Geometry check sheet. Reference: the model listing, model coordinates, mm. Coordinates: 2 decimals unless noted, no trailing zeros. Order: outer loops, then holes, each group sorted by start corner. A loop starts at its lowest first (then second) coordinate and runs counter-clockwise, first axis right, second up. Notation, with made-up numbers: M -15.75,53.5 L -1.75,53.5 A12 ccw -1.75,65.5 Z; hole C -3.75,36.25 d5. An arc over 180 degrees is marked long. One line per item, written item: value. Start each with the question number.
1) Go/stop test with flat-tipped pins: P1, Ø1.5, axis at y = 20, z = 3, coming from the +X side; P2, Ø1.5, axis at y = 99, z = 2, coming from the +X side (3 decimals); P3, Ø4.5, axis at x = -106, y = -70.5, coming from the +Z side. Record where each tip stops, or that it passes through.
2) Sectioned sample at D-D, the plane y = -207. Enter the section's corners in (x, z), then the cut area to 3 significant figures.
3) Thickness scan on L1, parallel to X at y = 81.5, z = 0.5; L2, parallel to Y at x = -1, z = 3.15; L3, parallel to X at y = -286.75, z = 1.15. Record the ranges inside material, lowest first. Write a range as from..to.
4) Sectioned sample at A-A, the plane y = -123. Enter the section's corners in (x, z).
5) Sectioned sample at C-C, the plane x = -61.5. Enter the section's corners in (y, z).
6) Sectioned sample at B-B, the plane z = 1.75. State how many separate pieces and enclosed holes the cut face has, then the cut area to 3 significant figures.
```python
from build123d import *

# Parameters (mm, degrees)
SKETCH1_R           = 2.75
BOSS_EXTRUDE1_DEPTH = 5
SKETCH2_R           = 3.25
BOSS_EXTRUDE2_DEPTH = 5
SKETCH3_R           = 2.75
BOSS_EXTRUDE3_DEPTH = 5
SKETCH4_R           = 3.25
BOSS_EXTRUDE4_DEPTH = 5
SKETCH5_R           = 2.75
BOSS_EXTRUDE5_DEPTH = 5
SKETCH6_R           = 3.25
BOSS_EXTRUDE6_DEPTH = 5


with BuildPart() as part:
    # Sketch1 → Boss-Extrude1 (new body)
    with BuildSketch(Plane.XY):
        Polygon((0, 210), (0, 0), (230, 0), (285, 210), align=None)
        with Locations((104, 185.5)):
            Circle(SKETCH1_R, mode=Mode.SUBTRACT)
        with Locations((194, 176)):
            Circle(SKETCH1_R, mode=Mode.SUBTRACT)
        with Locations((108.5, 130)):
            Circle(SKETCH1_R, mode=Mode.SUBTRACT)
        with Locations((193.5, 112)):
            Circle(SKETCH1_R, mode=Mode.SUBTRACT)
        with Locations((138.5, 82.5)):
            Circle(SKETCH1_R, mode=Mode.SUBTRACT)
        with Locations((167.5, 79.5)):
            Circle(SKETCH1_R, mode=Mode.SUBTRACT)
        with Locations((40, 83)):
            Circle(SKETCH1_R, mode=Mode.SUBTRACT)
        with Locations((66, 79)):
            Circle(SKETCH1_R, mode=Mode.SUBTRACT)
    extrude(amount=BOSS_EXTRUDE1_DEPTH)

    # Sketch2 → Boss-Extrude2 (add)
    with BuildSketch(Plane.XY):
        with BuildLine():
            Line((-202.121956495, 0), (0, 0))
            Line((0, 0), (0, 210))
            Line((0, 210), (-290, 210))
            Line((-290, 210), (-230, 0))
            Line((-230, 0), (-208.306614933, 0))
            ThreePointArc((-208.306614933, 0), (-205.214285714, 2.25), (-202.121956495, 0))
        make_face()
        with Locations((-237, 115.5)):
            Circle(SKETCH2_R, mode=Mode.SUBTRACT)
    extrude(amount=BOSS_EXTRUDE2_DEPTH)

    # Sketch3 → Boss-Extrude3 (add)
    with BuildSketch(Plane.XY):
        with BuildLine():
            Line((-208.306614933, 0), (-230, 0))
            Line((-230, 0), (-170, -210))
            Line((-170, -210), (-68.5, -210))
            Line((-68.5, -210), (-68.5, -81.5))
            Line((-68.5, -81.5), (0, -81.5))
            Line((0, -81.5), (0, -25.304886114))
            ThreePointArc((0, -25.304886114), (-4.25, -23), (0, -20.695113886))
            Line((0, -20.695113886), (0, 0))
            Line((0, 0), (-202.121956495, 0))
            ThreePointArc((-202.121956495, 0), (-202.003945393, -0.493823135), (-201.964285714, -1))
            ThreePointArc((-201.964285714, -1), (-205.720462579, -4.210340322), (-208.306614933, 0))
        make_face()
        with Locations((-106, -70.5)):
            Circle(SKETCH3_R, mode=Mode.SUBTRACT)
        with Locations((-93.5, -65.5)):
            Circle(SKETCH3_R, mode=Mode.SUBTRACT)
        with Locations((-4, -68.75)):
            Circle(SKETCH3_R, mode=Mode.SUBTRACT)
        with Locations((-105.75, -23.5)):
            Circle(SKETCH3_R, mode=Mode.SUBTRACT)
        with Locations((-93.25, -18.5)):
            Circle(SKETCH3_R, mode=Mode.SUBTRACT)
    extrude(amount=BOSS_EXTRUDE3_DEPTH)

    # Sketch4 → Boss-Extrude4 (add)
    with BuildSketch(Plane.XY):
        Polygon((-170, -210), (-126.5, -362.25), (-68.5, -362.25), (-68.5, -210), align=None)
        with Locations((-93, -347.75)):
            Circle(SKETCH4_R, mode=Mode.SUBTRACT)
        with Locations((-91, -282.25)):
            Circle(SKETCH4_R, mode=Mode.SUBTRACT)
    extrude(amount=BOSS_EXTRUDE4_DEPTH)

    # Sketch5 → Boss-Extrude5 (add)
    with BuildSketch(Plane.XY):
        with BuildLine():
            Line((0, -25.304886114), (0, -81.5))
            Line((0, -81.5), (75, -81.5))
            Line((75, -81.5), (75, -210))
            Line((75, -210), (175, -210))
            Line((175, -210), (230, 0))
            Line((230, 0), (0, 0))
            Line((0, 0), (0, -20.695113886))
            ThreePointArc((0, -20.695113886), (0.917384951, -21.68898894), (1.25, -23))
            ThreePointArc((1.25, -23), (0.917384951, -24.31101106), (0, -25.304886114))
        make_face()
        with Locations((11.5, -66.5)):
            Circle(SKETCH5_R, mode=Mode.SUBTRACT)
        with Locations((10.5, -20.5)):
            Circle(SKETCH5_R, mode=Mode.SUBTRACT)
        with Locations((165.5, -29.5)):
            Circle(SKETCH5_R, mode=Mode.SUBTRACT)
        with Locations((141, -24)):
            Circle(SKETCH5_R, mode=Mode.SUBTRACT)
    extrude(amount=BOSS_EXTRUDE5_DEPTH)

    # Sketch6 → Boss-Extrude6 (add)
    with BuildSketch(Plane.XY):
        Polygon((75, -210), (75, -362.25), (135.125, -362.25), (175, -210), align=None)
        with Locations((97.75, -350.75)):
            Circle(SKETCH6_R, mode=Mode.SUBTRACT)
        with Locations((97, -286.75)):
            Circle(SKETCH6_R, mode=Mode.SUBTRACT)
    extrude(amount=BOSS_EXTRUDE6_DEPTH)


solid = part.part
```
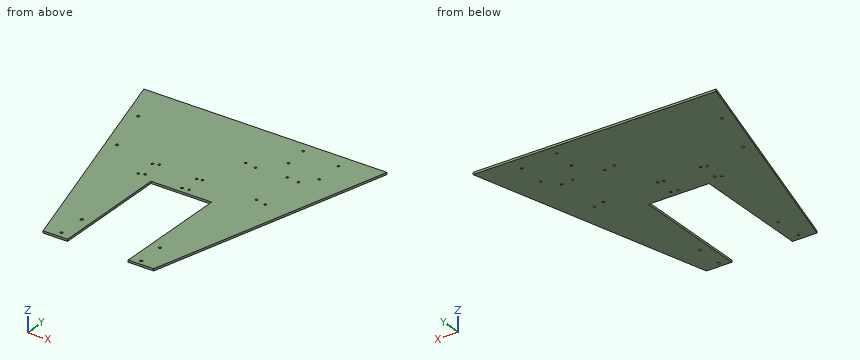
Final values:
1. P1: stops at x = 235.43
1. P2: stops at x = 256.125
1. P3: passes through
2. outline: M -170.86,0 L -68.5,0 L -68.5,5 L -170.86,5 Z; M 75,0 L 175.79,0 L 175.79,5 L 75,5 Z
2. area: 1,020 mm^2
3. L1: x = -253.29..37.7, 42.3..64.85, 67.15..135.94, 141.06..165.61, 169.39..251.35
3. L2: y = -81.5..-25.7, -20.3..210
3. L3: x = -148.07..-68.5, 75..93.75, 100.25..154.9
4. outline: M -194.86,0 L -68.5,0 L -68.5,5 L -194.86,5 Z; M 75,0 L 197.79,0 L 197.79,5 L 75,5 Z
5. outline: M -81.5,0 L 210,0 L 210,5 L -81.5,5 Z
6. separate pieces: 1
6. enclosed holes: 24
6. area: 198,000 mm^2
